from build123d import *

# Parameters (mm, degrees)
SZKIC1_R                        = 50
SZKIC1_R_2                      = 26
DODANIE_WYCI_GNI_CIE1_DEPTH     = 5
SZKIC3_R                        = 3.5
WYTNIJ_WYCI_GNI_CIE4_DEPTH      = 1
WYTNIJ_WYCI_GNI_CIE4_DEPTH_BACK = 6


with BuildPart() as part:
    # Szkic1 → Dodanie-wyciągnięcie1 (new body)
    with BuildSketch(Plane.XY):
        Circle(SZKIC1_R)
        Circle(SZKIC1_R_2, mode=Mode.SUBTRACT)
    extrude(amount=DODANIE_WYCI_GNI_CIE1_DEPTH)

    # Szkic3 → Wytnij-wyciągnięcie4 (cut, two sides)
    with BuildSketch(Plane.XY.offset(5)) as wytnij_wyci_gni_cie4_sk:
        with Locations((0, 42.5)):
            Circle(SZKIC3_R)
        with Locations((36.806079661, -21.25)):
            Circle(SZKIC3_R)
        with Locations((-36.806079661, -21.25)):
            Circle(SZKIC3_R)
    extrude(amount=WYTNIJ_WYCI_GNI_CIE4_DEPTH, mode=Mode.SUBTRACT)
    extrude(wytnij_wyci_gni_cie4_sk.sketch, amount=-WYTNIJ_WYCI_GNI_CIE4_DEPTH_BACK, mode=Mode.SUBTRACT)


solid = part.part
Read the model definition and answer for the solid it produces. Units are mm, in the model's axes. Round coordinates to 2 decimals unless told otherwise and drop trailing zeros. Loops run counter-clockwise (first coordinate to the right, second up) from the corner with the lowest first, then second, coordinate; pieces in that order, holes last.
Q1. Determine the mould class of faces 1 (the face through (-37.26, -17.78, 2.54)), 2 (the face through (22, -22, 5)), 3 (the face through (38.69, -18.3, 2.54)), 4 (the face through (47.69, 15.02, 2.46)) for opening direction X: released by +X, released by -X, zero draft, split by the parting line, or undercut.
Q2. Each of these flat-tipped pins is pushed along its axis until it touches: pin 1 (12 mm diameter, centred on x = 23, y = 25, fed in from -Z); pin 2 (1.5 mm diameter, centred on x = 33, z = 2.5, fed in from -Y); pin 3 (3 mm diameter, centred on y = -23, z = 2.5, fed in from -X); pin 4 (1 mm diameter, centred on y = -10, z = 2.5, fed in from +X). Where does it stop, or does it pass through?
Q3. Section C-C on z = 2.8 is taken. Write down the section's boundary in (x, y), and give its area (3 significant figures).
Q4. Section D-D on x = -36.5 is taken. Write down the section's boundary in (y, z).
Q5. Section B-B on x = 0 is taken. Write down the section's boundary in (y, z).
Q6. Section A-A on y = 0 is taken. Write down the section's boundary in (x, z).
Q7. Consider probe 1 along Y at (x, z) = (0, 2.45); probe 2 along X at (y, z) = (1, 3.05); probe 3 along Y at (x, z) = (18.5, 2.75). Determine where each line is inside the solid, lowest interval first.
Output:
1. face 1: undercut
1. face 2: zero draft
1. face 3: undercut
1. face 4: split by the parting line
2. pin 1: stops at z = 0
2. pin 2: stops at y = -38.21
2. pin 3: stops at x = -45.14
2. pin 4: stops at x = 49.09
3. outline: circle Ø100 at (0, 0); hole circle Ø7 at (-36.81, -21.25); hole circle Ø52 at (0, 0); hole circle Ø7 at (0, 42.5); hole circle Ø7 at (36.81, -21.25)
3. area: 5,610 mm2
4. outline: (-34.17, 0) - (-24.74, 0) - (-24.74, 5) - (-34.17, 5) - close; (-17.76, 0) - (34.17, 0) - (34.17, 5) - (-17.76, 5) - close
5. outline: (-50, 0) - (-26, 0) - (-26, 5) - (-50, 5) - close; (26, 0) - (39, 0) - (39, 5) - (26, 5) - close; (46, 0) - (50, 0) - (50, 5) - (46, 5) - close
6. outline: (-50, 0) - (-26, 0) - (-26, 5) - (-50, 5) - close; (26, 0) - (50, 0) - (50, 5) - (26, 5) - close
7. probe 1: y = -50 to -26, 26 to 39, 46 to 50
7. probe 2: x = -49.99 to -25.98, 25.98 to 49.99
7. probe 3: y = -46.45 to -18.27, 18.27 to 46.45
